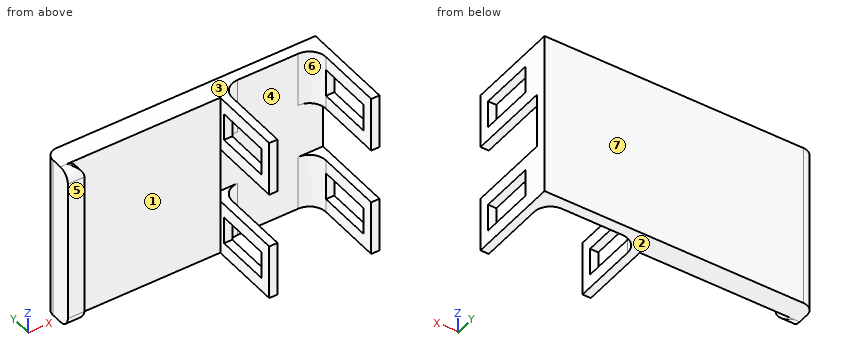
Autodesk Inventor part; units mm, degrees
ref_plane "YZ Plane" through (0, 0, 0) normal (1, 0, 0) x (0, 1, 0)
ref_plane "XZ Plane" through (0, 0, 0) normal (0, 1, 0) x (-1, 0, 0)
ref_plane "XY Plane" through (0, 0, 0) normal (0, 0, 1) x (1, 0, 0)
sketch "スケッチ1" plane through (0, 0, 0) normal (0, 0, 1) x (1, 0, 0)
  line L0 (-10, 17) -> (0, 17)
  line L1 (0, 17) -> (0, 15)
  line L2 (0, 15) -> (-10, 15)
  line L3 (-10, 15) -> (-10, 17)
  line L4 (0, -3.4) -> (0, 20.4)
  point P0 (0, 0)
  dimension "d0" = 10
  dimension "d1" = 2
  dimension "d2" = 15
extrude "押し出し1" add sketch "スケッチ1" along normal blind 5
sketch "スケッチ2" plane through (0, 0, 5) normal (0, 0, 1) x (1, 0, 0)
  line L0 (0, 17) -> (-10, 17)
  line L1 (-10, 17) -> (-8.5, 17)
  line L2 (-8.5, 17) -> (-8.5, 0)
  line L3 (-8.5, 0) -> (-10, 0)
  line L4 (-10, 0) -> (-10, 17)
  line L5 (-10, 15) -> (0, 15)
  line L6 (0, 15) -> (0, 17)
  line L7 (0, 17) -> (-10, 17)
  line L8 (-10, 17) -> (-10, 15)
  point P0 (0, 0)
  point P1 (-8.5, 15)
  dimension "d5" = 1.5
extrude "押し出し2" add sketch "スケッチ2" along normal blind 10
sketch "スケッチ3" plane through (-8.5, 0, 5) normal (1, 0, 0) x (0, 0, -1)
  line L0 (-7.5, 12) -> (-2.5, 12)
  line L1 (-2.5, 12) -> (-2.5, 2)
  line L2 (-2.5, 2) -> (-7.5, 2)
  line L3 (-7.5, 2) -> (-7.5, 12)
  line L4 (0, 0) -> (-10, 0)
  line L5 (0, 15) -> (-10, 15)
  point P0 (5, 0)
  point P1 (-5, 2)
  point P2 (-5, 0)
  dimension "d8" = 2
  dimension "d9" = 5
  dimension "d13" = 3
extrude "押し出し3" cut sketch "スケッチ3" against normal through all
fillet "フィレット1" radius 3 1 edges at (-8.5, 15, 10)
mirror "ミラー1" about plane through (0, 15, 0) normal (1, 0, 0)
mirror "ミラー2" about plane through (-5, 16, 0) normal (0, 0, -1)
sketch "スケッチ4" plane through (0, 0, 15) normal (0, 0, 1) x (1, 0, 0)
  line L0 (-10, 17) -> (-10, 0)
  line L1 (-10, 17) -> (-39, 17)
  line L2 (-39, 17) -> (-39, 13)
  line L3 (-39, 13) -> (-10, 13)
  line L4 (-10, 13) -> (-10, 17)
  line L5 (-39, 17) -> (-36, 17)
  line L6 (-36, 17) -> (-36, 11)
  line L7 (-36, 11) -> (-39, 11)
  line L8 (-39, 11) -> (-39, 17)
  point P0 (0, 0)
  point P1 (-36, 13)
  dimension "d14" = 4
  dimension "d15" = 3
  dimension "d16" = 26
  dimension "d17" = 6
extrude "押し出し4" add sketch "スケッチ4" against normal up to surface (30 mm away)
fillet "フィレット2" radius 2 1 edges at (-39, 17, 0)
fillet "フィレット3" radius 2 4 edges at (-36, 12, 15) (-37.5, 11, 15) (-37.5, 11, -15) (-36, 12, -15)
properties part number "connetcor_female_cover"
The listing builds one solid part. Answer for the finished solid, in the listing's coordinates (mm). Face numbers are marked on the shaded views. A direction names the side the tool comes from. Round coordinates to 2 decimals unless told otherwise and drop trailing zeros. Write each loop counter-clockwise with the first axis right and the second up, starting at its lowest first coordinate (ties: lowest second). Pieces come first, ordered by that corner, then holes. Notation, with made-up numbers: (33, -29.5) - (52, -29.5) arc R10 cw to (52, -13.5) - close; hole circle Ø5 at (1.5, -35). An arc over 180 degrees is marked (long way). Use a Markdown table: item, result. Add a question column.
1. Flat-ended cylindrical pins translate along their axes: P1, Ø1.6, axis at y = 13.5, z = 1.5, coming from the +X side; P2, Ø4, axis at y = 4.5, z = -4.5, coming from the -X side; P3, Ø4, axis at x = -5, z = 1, coming from the -Y side. Find the tip coordinate at first contact, or state that the pin passes through.
2. The part is cut by section D-D (x = -5). Write down the section's boundary in (y, z), and give its area (3 significant figures).
3. The part is cut by section C-C (z = -0.25). Write down the section's boundary in (x, y), and give its area (3 significant figures).
4. The part is cut by section A-A (y = 7). Give the number of separate pieces and of enclosed holes in the cut face, and give its area (3 significant figures).
5. A tool of negligible diameter and unlimited length cuts with its end or side. For the marked faces 5, 6 and 7, from which of +Z, -Z, +X, -X, +Y, -Y can it reach the whole face along a straight path? Write none if from no direction.
6. Consider line 1 (X direction, y = 3.75, z = -13.5); line 2 (X direction, y = 12.75, z = 9.5); line 3 (Y direction, x = -9.5, z = 9). Determine where each line is inside the solid, lowest interval first.
7. For a pull along Z with two mould halves and no side action, classify the marked faces 1, 2, 3 and 4 as +Z half, -Z half, draft (parallel to the pull), parting line (faces both ways), or undercut.
Reported:
| question | item | result |
|---|---|---|
| 1 | P1 | x = -10 |
| 1 | P2 | x = -10 |
| 1 | P3 | y = 15 |
| 2 | outline | (15, -15) - (17, -15) - (17, 15) - (15, 15) - close |
| 2 | area | 60.0 mm^2 |
| 3 | outline | (-39, 11) - (-36, 11) - (-36, 13) - (-10, 13) - (-10, 15) - (10, 15) - (10, 17) - (-37, 17) arc R2 ccw to (-39, 15) - close |
| 3 | area | 161 mm^2 |
| 4 | separate pieces | 8 |
| 4 | enclosed holes | 0 |
| 4 | area | 30.0 mm^2 |
| 5 | face 5 | +Z, -Z, -X, -Y |
| 5 | face 6 | +Z, -Z, -Y |
| 5 | face 7 | +Z, -Z, +X, -X, +Y |
| 6 | line 1 | -10 to -8.5, 8.5 to 10 |
| 6 | line 2 | -39 to -36, -10 to -8.4, 8.4 to 10 |
| 6 | line 3 | 0 to 2, 12 to 17 |
| 7 | face 1 | draft |
| 7 | face 2 | -Z half |
| 7 | face 3 | +Z half |
| 7 | face 4 | undercut |
